```python
from build123d import *

# Parameters (mm, degrees)
SKETCH_W        = 40
SKETCH_H        = 70
SKETCH_R        = 5.5
SKETCH_W_2      = 16
SKETCH_H_2      = 21.5
PAD_DEPTH       = 2
SKETCH001_W     = 5.6
SKETCH001_H     = 5.6
SKETCH001_W_2   = 16
SKETCH001_H_2   = 21.5
PAD001_DEPTH    = 6.5
SKETCH002_R     = 1.625
PAD002_DEPTH    = 2.5
SKETCH003_W     = 16
SKETCH003_H     = 1
SKETCH003_W_2   = 18
POCKET_DEPTH    = 1.5
SKETCH004_W     = 5.3
SKETCH004_H     = 4.3
POCKET001_DEPTH = 2.001
SKETCH005_R     = 1.6
SKETCH005_W     = 8.4
SKETCH005_H     = 1
PAD003_DEPTH    = 1.75
SKETCH006_W     = 36
SKETCH006_H     = 66
SKETCH006_W_2   = 34.4
SKETCH006_H_2   = 64.4
PAD004_DEPTH    = 2.5


with BuildPart() as part:
    # Sketch → Pad (new body)
    with BuildSketch(Plane.XY):
        Rectangle(SKETCH_W, SKETCH_H)
        with Locations((0, 23)):
            Circle(SKETCH_R, mode=Mode.SUBTRACT)
        Rectangle(SKETCH_W_2, SKETCH_H_2, mode=Mode.SUBTRACT)
    extrude(amount=PAD_DEPTH)

    # Sketch001 (on Face11 of Pad) → Pad001 (join)
    with BuildSketch(Plane.XY.offset(2)):
        with Locations((-8.5, -18.75)):
            Rectangle(SKETCH001_W, SKETCH001_H)
        with Locations((8.5, -18.75)):
            Rectangle(SKETCH001_W, SKETCH001_H)
        with BuildLine():
            Line((-8, -11.75), (8, -11.75))
            ThreePointArc((9, -10.75), (8.707107, -11.457107), (8, -11.75))
            Line((9, -10.75), (9, 10.75))
            ThreePointArc((8, 11.75), (8.707107, 11.457107), (9, 10.75))
            Line((8, 11.75), (0.8, 11.75))
            ThreePointArc((0.8, 11.75), (0, 14.243313), (-0.8, 11.75))
            Line((-0.8, 11.75), (-8, 11.75))
            ThreePointArc((-9, 10.75), (-8.707107, 11.457107), (-8, 11.75))
            Line((-9, 10.75), (-9, -10.75))
            ThreePointArc((-8, -11.75), (-8.707107, -11.457107), (-9, -10.75))
        make_face()
        Rectangle(SKETCH001_W_2, SKETCH001_H_2, mode=Mode.SUBTRACT)
    extrude(amount=PAD001_DEPTH)

    # Sketch002 (on Face34 of Pad001) → Pad002 (join)
    with BuildSketch(Plane.XY.offset(8.5)):
        with Locations((-8.5, -18.75)):
            Circle(SKETCH002_R)
        with Locations((8.5, -18.75)):
            Circle(SKETCH002_R)
    extrude(amount=PAD002_DEPTH)

    # Sketch003 (on Face35 of Pad002) → Pocket (cut)
    with BuildSketch(Plane.XY.offset(8.5)):
        with Locations((0, 11.25)):
            Rectangle(SKETCH003_W, SKETCH003_H)
        with Locations((0, -11.25)):
            Rectangle(SKETCH003_W_2, SKETCH003_H)
    extrude(amount=-POCKET_DEPTH, mode=Mode.SUBTRACT)

    # Sketch004 (on Face5 of Pocket) → Pocket001 (cut, through all)
    with BuildSketch(Plane.XY.offset(2)):
        with Locations((12, 23)):
            Rectangle(SKETCH004_W, SKETCH004_H)
    extrude(amount=-POCKET001_DEPTH, mode=Mode.SUBTRACT)

    # Sketch005 (on Face5 of Pocket001) → Pad003 (join)
    with BuildSketch(Plane.XY.offset(2)):
        with Locations((12, 17.85)):
            Circle(SKETCH005_R)
        with Locations((12, 14.75)):
            Rectangle(SKETCH005_W, SKETCH005_H)
    extrude(amount=PAD003_DEPTH)

    # Sketch006 (on Face5 of Pad003) → Pad004 (join)
    with BuildSketch(Plane.XY.offset(2)):
        Rectangle(SKETCH006_W, SKETCH006_H)
        Rectangle(SKETCH006_W_2, SKETCH006_H_2, mode=Mode.SUBTRACT)
    extrude(amount=PAD004_DEPTH)


solid = part.part
```
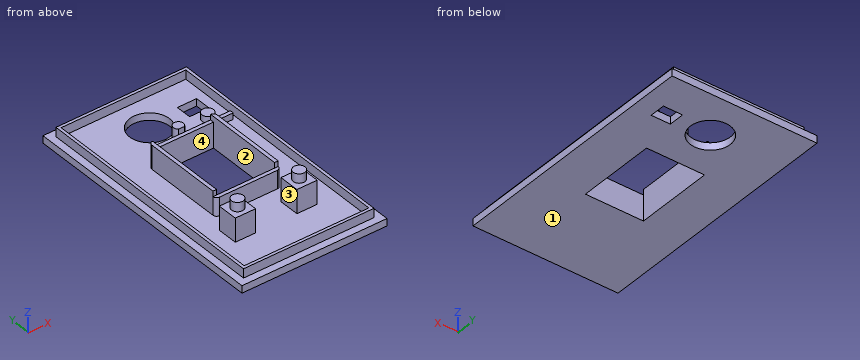
Build history of the part. All positions in model axes, mm. Face numbers are marked on the shaded views. A direction names the side the tool comes from. Give positions to 0.01 mm unless a question says otherwise; leave off trailing zeros. Order: outer loops, then holes, each group sorted by start corner. A loop starts at its lowest first (then second) coordinate and runs counter-clockwise, first axis right, second up. Notation, with made-up numbers: M 20,-29 L 63,-29 A10 ccw 63,-13 Z; hole C 67.5,32.5 d10. An arc over 180 degrees is marked long. Return JSON: item names as keys, results as strings.
Q1. Band-saw the part on D-D (z = 10). Give the cut face in (x, y) (3 decimals), then the cut area to 3 significant figures.
Answer list:
{"outline": "C -8.5,-18.75 d3.25; C 8.5,-18.75 d3.25", "area": "16.6 mm^2"}
Q2. Wall check: probe 1 along Y at (x, z) = (0, 0.6); probe 2 along Y at (x, z) = (3, 4); probe 3 along Y at (x, z) = (-10.5, 4). Give the ranges that are in metal, low to high. Write a range as from..to.
Answer list:
{"probe 1": "y = -35..-10.75, 10.75..17.5, 28.5..35", "probe 2": "y = -33..-32.2, -11.75..-10.75, 10.75..11.75, 32.2..33", "probe 3": "y = -33..-32.2, -21.55..-15.95, 32.2..33"}
Q3. 3-axis set-ups, long thin cutter, end or side, ignore diameter. For the marked faces 3 and 4: which of +Z, -Z, +X, -X, +Y, -Y reach the whole face in a straight line?
Answer list:
{"face 3": "+Z", "face 4": "+Z, -Z"}
Q4. Flat gauge pins, fed straight in: pin 1 (6 mm diameter, centred on x = -9, y = -12, fed in from -Z); pin 2 (0.5 mm diameter, centred on x = 14, y = 14.5, fed in from +Z); pin 3 (0.8 mm diameter, centred on x = 6, z = 3, fed in from -Y); pin 4 (3 mm diameter, centred on x = -8.5, z = 6.5, fed in from +Y). Where does each tip first touch, or does it go through?
Answer list:
{"pin 1": "stops at z = 0", "pin 2": "stops at z = 3.75", "pin 3": "stops at y = -33", "pin 4": "stops at y = 11.75"}
Q5. Band-saw the part on B-B (x = 0). Give the cut face in (y, z), then the cut area to 3 significant figures.
Answer list:
{"outline": "M -35,0 L -10.75,0 L -10.75,7 L -11.75,7 L -11.75,2 L -32.2,2 L -32.2,4.5 L -33,4.5 L -33,2 L -35,2 Z; M 10.75,0 L 17.5,0 L 17.5,2 L 14.24,2 L 14.24,8.5 L 11.75,8.5 L 11.75,7 L 10.75,7 Z; M 28.5,0 L 35,0 L 35,2 L 33,2 L 33,4.5 L 32.2,4.5 L 32.2,2 L 28.5,2 Z", "area": "105 mm^2"}
Q6. Band-saw the part on C-C (y = 23). Give the cut face in (x, z).
Answer list:
{"outline": "M -20,0 L -5.5,0 L -5.5,2 L -17.2,2 L -17.2,4.5 L -18,4.5 L -18,2 L -20,2 Z; M 5.5,0 L 9.35,0 L 9.35,2 L 5.5,2 Z; M 14.65,0 L 20,0 L 20,2 L 18,2 L 18,4.5 L 17.2,4.5 L 17.2,2 L 14.65,2 Z"}
Q7. Band-saw the part on A-A (x = 12). Give the cut face in (y, z), then the cut area to 3 significant figures.
Answer list:
{"outline": "M -35,0 L 20.85,0 L 20.85,2 L 19.45,2 L 19.45,3.75 L 16.25,3.75 L 16.25,2 L 15.25,2 L 15.25,3.75 L 14.25,3.75 L 14.25,2 L -32.2,2 L -32.2,4.5 L -33,4.5 L -33,2 L -35,2 Z; M 25.15,0 L 35,0 L 35,2 L 33,2 L 33,4.5 L 32.2,4.5 L 32.2,2 L 25.15,2 Z", "area": "143 mm^2"}
Q8. Two-plate mould, pull along X, no slides. Class the marked faces 1 and 2: pulls with the +X half, pulls with the -X half, needs draft (parallel to the pull), parting line crosses it, or undercut.
Answer list:
{"face 1": "needs draft", "face 2": "undercut"}
